Part model, mm, in its own coordinate system. Face numbers are marked on the shaded views. A direction names the side the tool comes from. Round coordinates to 2 decimals unless told otherwise and drop trailing zeros. Write each loop counter-clockwise with the first axis right and the second up, starting at its lowest first coordinate (ties: lowest second). Pieces come first, ordered by that corner, then holes. Notation, with made-up numbers: M 53,48.5 L 81,48.5 A22 cw 81,81.5 Z; hole C 82,40.25 d3. An arc over 180 degrees is marked long. Use a Markdown table: item, result. Add a question column.
1) Slice it at C-C on y = 50. Write the cut outline in (x, z).
2) Two-plate mould, pull along X, no slides. Class the marked faces 4, 5, 6 and 7: released by +X, released by -X, zero draft, split by the parting line, or undercut.
3) Slice it at A-A on z = 1.5. Write the cut outline in (x, y).
4) Which spindle directions (+Z, -Z, +X, -X, +Y, -Y) get a long thin tool onto all of the face, cutting with end or side? Do the marked faces 1, 2 and 3. Say none if no direction does.
5) Drop flat-ended pins along their axis: P1, Ø2.5, axis at y = 9, z = 7.5, coming from the -X side; P2, Ø0.9, axis at x = 5, y = 20, coming from the +Z side. Give the stop position or say it passes through.
6) Slice it at B-B on x = 5. Write the cut outline in (y, z).
7) Slice it at D-D on x = 21. Write the cut outline in (y, z).
8) Wall check: probe 1 along Y at (x, z) = (5, 13.25); probe 2 along Y at (x, z) = (13.5, 7.75); probe 3 along Z at (x, y) = (29, 28.5). Give the ranges that are in metal, low to high.
```python
from build123d import *

# Parameters (mm, degrees)
ESQUISSE1_W             = 50
ESQUISSE1_H             = 60
BOSS_EXTRU_1_DEPTH      = 15
ESQUISSE2_R             = 4.25
ESQUISSE2_R_2           = 5
ENL_V_MAT_EXTRU_1_DEPTH = 8
ESQUISSE4_W             = 2.260138716
ESQUISSE4_H             = 60
ENL_V_MAT_EXTRU_2_DEPTH = 80.529868603
ESQUISSE5_R             = 4
ENL_V_MAT_EXTRU_3_DEPTH = 8
ESQUISSE6_W             = 47.739861284
ESQUISSE6_H             = 4.016031869
ENL_V_MAT_EXTRU_4_DEPTH = 79.128703787
CONG_1_R                = 3
ESQUISSE7_R             = 1.5
ENL_V_MAT_EXTRU_5_DEPTH = 5


with BuildPart() as part:
    # Esquisse1 → Boss.-Extru.1 (new body)
    with BuildSketch(Plane.XY):
        with Locations((25, 30)):
            Rectangle(ESQUISSE1_W, ESQUISSE1_H)
    extrude(amount=BOSS_EXTRU_1_DEPTH)

    # Esquisse2 → Enlèv. mat.-Extru.1 (cut)
    with BuildSketch(Plane.XY):
        with Locations((10, 36.14)):
            Circle(ESQUISSE2_R)
        with Locations((10, 19.84)):
            Circle(ESQUISSE2_R)
        with Locations((24.644968419, 27.99)):
            Circle(ESQUISSE2_R_2)
    extrude(amount=ENL_V_MAT_EXTRU_1_DEPTH, mode=Mode.SUBTRACT)

    # Esquisse4 → Enlèv. mat.-Extru.2 (cut, through all)
    with BuildSketch(Plane.XY):
        with Locations((48.869930642, 30)):
            Rectangle(ESQUISSE4_W, ESQUISSE4_H)
    extrude(amount=ENL_V_MAT_EXTRU_2_DEPTH, mode=Mode.SUBTRACT)

    # Esquisse5 → Enlèv. mat.-Extru.3 (cut)
    with BuildSketch(Plane(origin=(0, 0, 0), x_dir=(0, 0, -1), z_dir=(1, 0, 0))):
        with Locations((-7.779969549, 8)):
            Circle(ESQUISSE5_R)
        with Locations((-7.779969549, 48)):
            Circle(ESQUISSE5_R)
    extrude(amount=ENL_V_MAT_EXTRU_3_DEPTH, mode=Mode.SUBTRACT)

    # Esquisse6 → Enlèv. mat.-Extru.4 (cut, through all)
    with BuildSketch(Plane(origin=(0, 0, 0), x_dir=(-1, 0, 0), z_dir=(0, 0, -1))):
        with Locations((-23.869930642, 57.991984066)):
            Rectangle(ESQUISSE6_W, ESQUISSE6_H)
    extrude(amount=-ENL_V_MAT_EXTRU_4_DEPTH, mode=Mode.SUBTRACT)

    # Congé1
    cong_1_edges = [part.edges().sort_by_distance(p)[0] for p in [
        (47.739861284, 0, 7.5),
        (47.739861284, 55.983968131, 7.5),
        (0, 55.983968131, 7.5),
        (0, 0, 7.5),
    ]]
    fillet(cong_1_edges, radius=CONG_1_R)

    # Esquisse7 → Enlèv. mat.-Extru.5 (cut)
    with BuildSketch(Plane.XY.offset(15)):
        with Locations((37.739861284, 45.983968131)):
            Circle(ESQUISSE7_R)
        with Locations((37.739861284, 10)):
            Circle(ESQUISSE7_R)
        with Locations((5, 20)):
            Circle(ESQUISSE7_R)
        with Locations((5, 35.983968131)):
            Circle(ESQUISSE7_R)
    extrude(amount=-ENL_V_MAT_EXTRU_5_DEPTH, mode=Mode.SUBTRACT)


solid = part.part
```
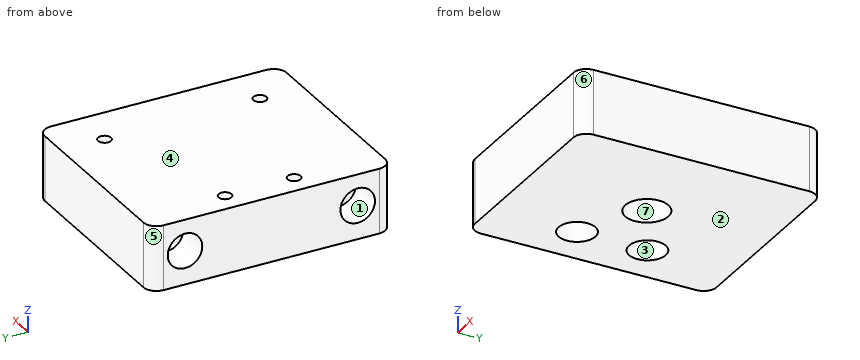
Entries:
| question | item | result |
|---|---|---|
| 1 | outline | M 0,0 L 47.74,0 L 47.74,15 L 0,15 L 0,11.24 L 8,11.24 L 8,4.32 L 0,4.32 Z |
| 2 | face 4 | zero draft |
| 2 | face 5 | released by -X |
| 2 | face 6 | released by +X |
| 2 | face 7 | undercut |
| 3 | outline | M 0,3 A3 ccw 3,0 L 44.74,0 A3 ccw 47.74,3 L 47.74,52.98 A3 ccw 44.74,55.98 L 3,55.98 A3 ccw 0,52.98 Z; hole C 10,19.84 d8.5; hole C 10,36.14 d8.5; hole C 24.64,27.99 d10 |
| 4 | face 1 | -X |
| 4 | face 2 | -Z, +X, -X, +Y, -Y |
| 4 | face 3 | -Z |
| 5 | P1 | stops at x = 8 |
| 5 | P2 | stops at z = 10 |
| 6 | outline | M 0,0 L 55.98,0 L 55.98,15 L 37.48,15 L 37.48,10 L 34.48,10 L 34.48,15 L 21.5,15 L 21.5,10 L 18.5,10 L 18.5,15 L 0,15 Z; hole C 8,7.78 d8; hole C 48,7.78 d8 |
| 7 | outline | M 0,0 L 24.57,0 L 24.57,8 L 31.41,8 L 31.41,0 L 55.98,0 L 55.98,15 L 0,15 Z |
| 8 | probe 1 | y = 0 to 18.5, 21.5 to 34.48, 37.48 to 55.98 |
| 8 | probe 2 | y = 0 to 17.43, 22.25 to 33.73, 38.55 to 55.98 |
| 8 | probe 3 | z = 8 to 15 |
